Verification items for the finished model (mm, model axes). Give positions to 0.01 mm unless a question says otherwise; leave off trailing zeros. Write each loop counter-clockwise with the first axis right and the second up, starting at its lowest first coordinate (ties: lowest second). Pieces come first, ordered by that corner, then holes. Notation, with made-up numbers: (56, -38) - (69, -38) arc R27 ccw to (69, -17) - close; hole circle Ø11 at (1.5, -19.5). An arc over 180 degrees is marked (long way). Put each result on its own line as item: value.
Autodesk Inventor part; units mm, degrees
ref_plane "YZ Plane" through (0, 0, 0) normal (1, 0, 0) x (0, 1, 0)
ref_plane "XZ Plane" through (0, 0, 0) normal (0, 1, 0) x (-1, 0, 0)
ref_plane "XY Plane" through (0, 0, 0) normal (0, 0, 1) x (1, 0, 0)
sketch3d "3D Sketch1"
sketch "Sketch8" plane through (0, 0, 0) normal (0, 1, 0) x (-1, 0, 0)
  arc A0 (-533.9727, 129.2939) -> (-533.9727, 72.7061) centre (-524, 101) ccw
  arc A1 (-533.9727, 129.2939) -> (-540.6211, 148.1565) centre (-537.2969, 138.7252) ccw
  arc A2 (-540.6211, 148.1565) -> (-540.6211, 53.8435) centre (-524, 101) ccw
  arc A3 (-540.6211, 53.8435) -> (-533.9727, 72.7061) centre (-537.2969, 63.2748) ccw
  circle A4 centre (-537.2969, 63.2748) radius 3
  circle A5 centre (-556.6482, 77.8001) radius 2.9994
  circle A6 centre (-564, 101) radius 3
  circle A7 centre (-556.6482, 124.1094) radius 2.9994
  circle A8 centre (-537.2969, 138.7252) radius 3
  point P0 (0, 0)
extrude "Extrusion1" add sketch "Sketch8" along normal blind 3
properties part number "pulsador_presion"
Q1. Section check C-C, the plane y = 2.25. Record the cut outline in (x, z), plus the area to 3 significant figures.
Answers follow:
outline: (533.97, 72.71) arc R10 ccw to (540.62, 53.84) arc R50 ccw to (540.62, 148.16) arc R10 ccw to (533.97, 129.29) arc R30 cw to start; hole circle Ø6 at (537.3, 63.27); hole circle Ø6 at (537.3, 138.73); hole circle Ø6 at (556.65, 77.8); hole circle Ø6 at (556.65, 124.11); hole circle Ø6 at (564, 101)
area: 2,140 mm2
Q2. Scan lines: line 1 along Z through (x, y) = (537, 0.55); line 2 along Z through (x, y) = (559, 1.8); line 3 along Z through (x, y) = (564, 1.6). Record each from-to range of solid material in increasing order.
Answers follow:
line 1: z = 53.28 to 60.29, 66.26 to 73.96, 128.04 to 135.74, 141.71 to 148.72
line 2: z = 65.29 to 75.94, 79.66 to 122.25, 125.97 to 136.71
line 3: z = 71 to 98, 104 to 131
Q3. Go/stop test with flat-tipped pins: pin 1 Ø1 at (x, y) = (535, 1) entering from +Z; pin 2 Ø1 at (y, z) = (2, 111.5) entering from -X; pin 3 Ø1 at (y, z) = (1.5, 103) entering from -X. Record where each tip stops, or that it passes through.
Answers follow:
pin 1: stops at z = 148.56
pin 2: stops at x = 551.91
pin 3: stops at x = 553.9
Q4. Release check for a two-part mould opening along X. For faces 1 (the face through (556, 3, 102)), 2 (the face through (553.996, 1.479, 100.483)), 3 (the face through (561.23, 1.48, 102.15)) record: released by +X, released by -X, zero draft, split by the parting line, or undercut.
Answers follow:
face 1: zero draft
face 2: released by -X
face 3: undercut
Q5. Section check D-D, the plane z = 85. Record the cut outline in (x, y), plus the area to 3 significant figures.
Answers follow:
outline: (549.38, 0) - (571.37, 0) - (571.37, 3) - (549.38, 3) - close
area: 66.0 mm2
Q6. Section check A-A, the plane z = 101. Record the cut outline in (x, y), plus the area to 3 significant figures.
Answers follow:
outline: (554, 0) - (561, 0) - (561, 3) - (554, 3) - close; (567, 0) - (574, 0) - (574, 3) - (567, 3) - close
area: 42.0 mm2
Q7. Section check B-B, the plane x = 530.5. Record the cut outline in (y, z).
Answers follow:
outline: (0, 55.94) - (3, 55.94) - (3, 70.61) - (0, 70.61) - close; (0, 131.39) - (3, 131.39) - (3, 146.06) - (0, 146.06) - close
